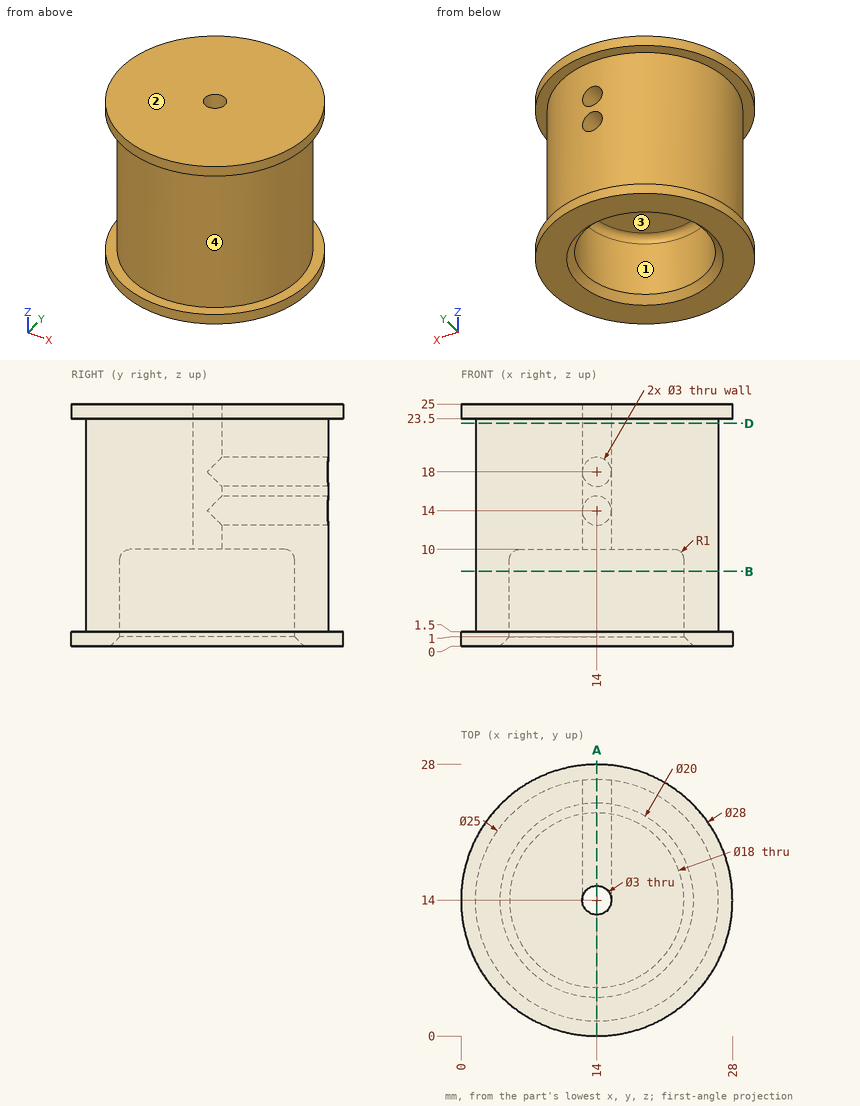
Input: dimensioned drawing with shaded views. Units: mm. Origin: part minimum x, y, z. Coordinates: 2 decimals unless noted, no trailing zeros. Order: outer loops, then holes, each group sorted by start corner. A loop starts at its lowest first (then second) coordinate and runs counter-clockwise, first axis right, second up. Notation, with made-up numbers: (86, -36) - (114, -36) arc R20 ccw to (114, -13) - close; hole circle Ø11 at (-19, 18). An arc over 180 degrees is marked (long way). Return JSON: item names as keys, results as strings. Group by question number.
1. Cut plane D-D (z = 23). Output: boundary loops of the cut face in (x, y).
2. Pull-direction query (Y, two-part tool) for the marked faces 1, 2, 3 and 4; classes: pulls with the +Y half, pulls with the -Y half, needs draft (parallel to the pull), parting line crosses it, or undercut.
3. Cut plane A-A (x = 14). Count the separate pieces of the cut face and the enclosed holes in it, plus the area to 3 significant figures.
4. Pin query (flat end, axial travel): pin 1 (13 mm diameter, centred on x = 12, y = 10.5, fed in from -Z); pin 2 (2.5 mm diameter, centred on x = 14, z = 18, fed in from +Y); pin 3 (6 mm diameter, centred on x = 16, z = 8, fed in from +Y); pin 4 (4 mm diameter, centred on y = 18.5, z = 6.5, fed in from +X). Return the tip coordinate at first contact, or that it passes through.
5. Cut plane B-B (z = 7.75). Output: boundary loops of the cut face in (x, y), plus the area to 3 significant figures.
6. Material intervals for line 1 along Z through (x, y) = (14, 20); line 2 along Z through (x, y) = (12, 26.5); line 3 along X through (y, z) = (13.5, 10.5), sorted ascending. Write a range as [from, to].
Resolved:
{
 "1": {"outline": "circle Ø25 at (14, 14); hole circle Ø3 at (14, 14)"},
 "2": {"face 1": "undercut", "face 2": "needs draft", "face 3": "undercut", "face 4": "parting line crosses it"},
 "3": {"separate pieces": "4", "enclosed holes": "0", "area": "342 mm²"},
 "4": {"pin 1": "stops at z = 0", "pin 2": "stops at y = 13.17", "pin 3": "stops at y = 26.5", "pin 4": "stops at x = 26.25"},
 "5": {"outline": "circle Ø25 at (14, 14); hole circle Ø18 at (14, 14)", "area": "236 mm²"},
 "6": {"line 1": "z = [10, 12.5], [15.5, 16.5], [19.5, 25]", "line 2": "z = [0, 1.5], [23.5, 25]", "line 3": "x = [1.51, 12.59], [15.41, 26.49]"}
}
